The listing builds one solid part. Answer for the finished solid, in the listing's coordinates (mm). A direction names the side the tool comes from. Give positions to 0.01 mm unless a question says otherwise; leave off trailing zeros. Order: outer loops, then holes, each group sorted by start corner. A loop starts at its lowest first (then second) coordinate and runs counter-clockwise, first axis right, second up. Notation, with made-up numbers: (9.25, 63.25) -> (36.25, 63.25) arc R21 ccw to (36.25, 69.25) -> close; hole circle Ø10 at (-8.5, -26.5). An arc over 180 degrees is marked (long way). One line per question, with ' | ' between items. Start each with the question number.
```python
from build123d import *

# Parameters (mm, degrees)
BASE_FLANGE_DEPTH               = 1.5875
EDGE_FLANGE1_STRIP_W            = 7.8232
EDGE_FLANGE1_STRIP_H            = 1.5875
EDGE_FLANGE1_STRIP_CUT_DEPTH    = 139.7
EDGE_FLANGE1_DEPTH              = 139.7
EDGE_FLANGE2_STRIP_W            = 7.8232
EDGE_FLANGE2_STRIP_H            = 1.5875
EDGE_FLANGE2_STRIP_CUT_DEPTH    = 139.7
EDGE_FLANGE2_DEPTH              = 139.7
EDGE_FLANGE3_STRIP_W            = 7.8232
EDGE_FLANGE3_STRIP_H            = 1.5875
EDGE_FLANGE3_STRIP_CUT_DEPTH    = 370.68125
EDGE_FLANGE3_DEPTH              = 370.68125
EDGE_FLANGE4_STRIP_W            = 7.8232
EDGE_FLANGE4_STRIP_H            = 1.5875
EDGE_FLANGE4_STRIP_CUT_DEPTH    = 370.68125
EDGE_FLANGE4_DEPTH              = 370.68125
SKETCH15_W                      = 20.4724
SKETCH15_H                      = 10.668
CUT_EXTRUDE1_DEPTH              = 458.107468491
SKETCH16_W                      = 17.653
SKETCH16_H                      = 13.081
CUT_EXTRUDE2_DEPTH              = 458.107468491
F_1_8_0_125_DIAMETER_HOLE1_D    = 3.175
LPATTERN2_COUNT                 = 2
LPATTERN2_PITCH                 = 24.9936
SKETCH20_W                      = 17.145
SKETCH20_H                      = 22.987
CUT_EXTRUDE4_DEPTH              = 458.107468491
F_40_0_098_DIAMETER_HOLE2_D     = 3.175
SKETCH31_W                      = 30.48
SKETCH31_H                      = 22.86
CUT_EXTRUDE5_DEPTH              = 458.107468491
F_40_0_098_DIAMETER_HOLE3_D     = 3.556
F_40_0_098_DIAMETER_HOLE4_D     = 3.556
F_40_0_098_DIAMETER_HOLE4_DEPTH = 1.5875
F_40_0_098_DIAMETER_HOLE4_TIP   = 1.068330181
FILLET1_R                       = 5.9436
SKETCH38_W                      = 20.4724
SKETCH38_H                      = 10.668
CUT_EXTRUDE6_DEPTH              = 2.54
LPATTERN3_COUNT                 = 2
LPATTERN3_PITCH                 = 32.4866
LPATTERN4_COUNT                 = 2
LPATTERN4_PITCH                 = 24.9936
LPATTERN5_COUNT                 = 2
LPATTERN5_PITCH                 = 32.4866
LPATTERN7_COUNT                 = 2
LPATTERN7_PITCH                 = 57.4802
LPATTERN8_COUNT                 = 2
LPATTERN8_PITCH                 = 88.9
SKETCH41_R                      = 4.7117
CUT_EXTRUDE7_DEPTH              = 2.54
SKETCH43_W                      = 7.7978
SKETCH43_H                      = 4.0132
CUT_EXTRUDE8_DEPTH              = 2.54
HOLE1_START                     = -15.0368
HOLE1_OUTLINE_R                 = 2.7051
HOLE1_DEPTH                     = 169.7736
LPATTERN9_COUNT                 = 3
LPATTERN9_PITCH                 = 177.8


# Read off the part's stored shape, not the designer's step: Hole1
# Sheet-metal steps are written as plain solids
with BuildPart() as part:
    # Sketch1 → Base-Flange (new body)
    with BuildSketch(Plane.XY):
        Polygon((0, 0), (28.832175, 0), (28.832175, -13.4493), (399.513425, -13.4493), (399.513425, 0), (428.3456, 0), (428.3456, 139.7), (399.513425, 139.7), (399.513425, 153.1493), (28.832175, 153.1493), (28.832175, 139.7), (0, 139.7), align=None)
    extrude(amount=BASE_FLANGE_DEPTH)

    # Edge-Flange1 strip (across the edge) → Edge-Flange1 strip cut (cut)
    with BuildSketch(Plane(origin=(428.3456, 0, 1.5875), x_dir=(-1, 0, 0), z_dir=(0, 1, 0))):
        with Locations((-3.175, -0.79375)):
            Rectangle(EDGE_FLANGE1_STRIP_W, EDGE_FLANGE1_STRIP_H)
    extrude(amount=EDGE_FLANGE1_STRIP_CUT_DEPTH, mode=Mode.SUBTRACT)

    # Edge-Flange1 section (across the edge) → Edge-Flange1 (add)
    with BuildSketch(Plane(origin=(428.3456, 0, 1.5875), x_dir=(-1, 0, 0), z_dir=(0, 1, 0))):
        with BuildLine():
            Line((-1.5875, 0.7366), (-1.5875, 12.7))
            Line((-1.5875, 12.7), (0, 12.7))
            Line((0, 12.7), (0, 0.7366))
            ThreePointArc((0, 0.7366), (0.215745145, 0.215745145), (0.7366, 0))
            Line((0.7366, 0), (0.7366, -1.5875))
            ThreePointArc((0.7366, -1.5875), (-0.90678687, -0.90678687), (-1.5875, 0.7366))
        make_face()
    extrude(amount=EDGE_FLANGE1_DEPTH)

    # Edge-Flange2 strip (across the edge) → Edge-Flange2 strip cut (cut)
    with BuildSketch(Plane(origin=(0, 139.7, 1.5875), x_dir=(1, 0, 0), z_dir=(0, -1, 0))):
        with Locations((-3.175, -0.79375)):
            Rectangle(EDGE_FLANGE2_STRIP_W, EDGE_FLANGE2_STRIP_H)
    extrude(amount=EDGE_FLANGE2_STRIP_CUT_DEPTH, mode=Mode.SUBTRACT)

    # Edge-Flange2 section (across the edge) → Edge-Flange2 (add)
    with BuildSketch(Plane(origin=(0, 139.7, 1.5875), x_dir=(1, 0, 0), z_dir=(0, -1, 0))):
        with BuildLine():
            Line((-1.5875, 0.7366), (-1.5875, 12.7))
            Line((-1.5875, 12.7), (0, 12.7))
            Line((0, 12.7), (0, 0.7366))
            ThreePointArc((0, 0.7366), (0.215745145, 0.215745145), (0.7366, 0))
            Line((0.7366, 0), (0.7366, -1.5875))
            ThreePointArc((0.7366, -1.5875), (-0.90678687, -0.90678687), (-1.5875, 0.7366))
        make_face()
    extrude(amount=EDGE_FLANGE2_DEPTH)

    # Edge-Flange3 strip (across the edge) → Edge-Flange3 strip cut (cut)
    with BuildSketch(Plane(origin=(399.513425, 153.1493, 1.5875), x_dir=(0, -1, 0), z_dir=(-1, 0, 0))):
        with Locations((-3.175, -0.79375)):
            Rectangle(EDGE_FLANGE3_STRIP_W, EDGE_FLANGE3_STRIP_H)
    extrude(amount=EDGE_FLANGE3_STRIP_CUT_DEPTH, mode=Mode.SUBTRACT)

    # Edge-Flange3 section (across the edge) → Edge-Flange3 (add)
    with BuildSketch(Plane(origin=(399.513425, 153.1493, 1.5875), x_dir=(0, -1, 0), z_dir=(-1, 0, 0))):
        with BuildLine():
            Line((-1.5875, 0.7366), (-1.5875, 12.7))
            Line((-1.5875, 12.7), (0, 12.7))
            Line((0, 12.7), (0, 0.7366))
            ThreePointArc((0, 0.7366), (0.215745145, 0.215745145), (0.7366, 0))
            Line((0.7366, 0), (0.7366, -1.5875))
            ThreePointArc((0.7366, -1.5875), (-0.90678687, -0.90678687), (-1.5875, 0.7366))
        make_face()
    extrude(amount=EDGE_FLANGE3_DEPTH)

    # Edge-Flange4 strip (across the edge) → Edge-Flange4 strip cut (cut)
    with BuildSketch(Plane(origin=(28.832175, -13.4493, 1.5875), x_dir=(0, 1, 0), z_dir=(1, 0, 0))):
        with Locations((-3.175, -0.79375)):
            Rectangle(EDGE_FLANGE4_STRIP_W, EDGE_FLANGE4_STRIP_H)
    extrude(amount=EDGE_FLANGE4_STRIP_CUT_DEPTH, mode=Mode.SUBTRACT)

    # Edge-Flange4 section (across the edge) → Edge-Flange4 (add)
    with BuildSketch(Plane(origin=(28.832175, -13.4493, 1.5875), x_dir=(0, 1, 0), z_dir=(1, 0, 0))):
        with BuildLine():
            Line((-1.5875, 0.7366), (-1.5875, 12.7))
            Line((-1.5875, 12.7), (0, 12.7))
            Line((0, 12.7), (0, 0.7366))
            ThreePointArc((0, 0.7366), (0.215745145, 0.215745145), (0.7366, 0))
            Line((0.7366, 0), (0.7366, -1.5875))
            ThreePointArc((0.7366, -1.5875), (-0.90678687, -0.90678687), (-1.5875, 0.7366))
        make_face()
    extrude(amount=EDGE_FLANGE4_DEPTH)

    # Sketch15 → Cut-Extrude1 (cut, through all)
    with BuildSketch(Plane.XY.offset(1.5875)):
        with Locations((74.4728, 119.6213)):
            Rectangle(SKETCH15_W, SKETCH15_H)
    extrude(amount=-CUT_EXTRUDE1_DEPTH, mode=Mode.SUBTRACT)

    # Sketch16 → Cut-Extrude2 (cut, through all)
    with BuildSketch(Plane.XY.offset(1.5875)):
        with Locations((105.8291, 119.6213)):
            Rectangle(SKETCH16_W, SKETCH16_H)
    extrude(amount=-CUT_EXTRUDE2_DEPTH, mode=Mode.SUBTRACT)

    # 1/8 (0.125) Diameter Hole1 (through all)
    with Locations(Plane.XY.offset(1.5875)):
        with Locations((61.976, 119.6213)):
            f_1_8_0_125_diameter_hole1 = Hole(F_1_8_0_125_DIAMETER_HOLE1_D / 2)

    # LPattern2: 1/8 (0.125) Diameter Hole1 ×2
    with Locations(*[(i * LPATTERN2_PITCH, 0, 0) for i in range(1, LPATTERN2_COUNT)]):
        add(f_1_8_0_125_diameter_hole1, mode=Mode.SUBTRACT)

    # Sketch20 → Cut-Extrude4 (cut, through all)
    with BuildSketch(Plane.XY.offset(1.5875)):
        with Locations((42.9641, 119.6213)):
            Rectangle(SKETCH20_W, SKETCH20_H)
    extrude(amount=-CUT_EXTRUDE4_DEPTH, mode=Mode.SUBTRACT)

    # #40 (0.098) Diameter Hole2 (through all)
    with Locations(Plane.XY.offset(1.5875)):
        with Locations((42.9641, 134.1247), (42.9641, 105.1179)):
            Hole(F_40_0_098_DIAMETER_HOLE2_D / 2)

    # Sketch31 → Cut-Extrude5 (cut, through all)
    with BuildSketch(Plane.XY.offset(1.5875)):
        with Locations((394.3731, 21.7932)):
            Rectangle(SKETCH31_W, SKETCH31_H)
    extrude(amount=-CUT_EXTRUDE5_DEPTH, mode=Mode.SUBTRACT)

    # #40 (0.098) Diameter Hole3 (through all)
    with Locations(Plane(origin=(374.3706, 21.7932, 1.5875), x_dir=(1, 0, 0), z_dir=(0, 0, 1))):
        with Locations((0, 0)):
            Hole(F_40_0_098_DIAMETER_HOLE3_D / 2)

    # #40 (0.098) Diameter Hole4
    with Locations(Plane.XY.offset(1.5875)):
        with Locations((414.3756, 21.7932)):
            Hole(F_40_0_098_DIAMETER_HOLE4_D / 2, depth=F_40_0_098_DIAMETER_HOLE4_DEPTH)
            with Locations((0, 0, -(F_40_0_098_DIAMETER_HOLE4_DEPTH + F_40_0_098_DIAMETER_HOLE4_TIP / 2))):  # 118° drill point
                Cone(0, F_40_0_098_DIAMETER_HOLE4_D / 2, F_40_0_098_DIAMETER_HOLE4_TIP, mode=Mode.SUBTRACT)

    # Fillet1
    fillet1_edges = [part.edges().sort_by_distance(p)[0] for p in [
        (379.1331, 10.3632, 0.79375),
        (379.1331, 33.2232, 0.79375),
        (409.6131, 33.2232, 0.79375),
        (409.6131, 10.3632, 0.79375),
    ]]
    fillet(fillet1_edges, radius=FILLET1_R)

    # Sketch38 → Cut-Extrude6 (cut)
    with BuildSketch(Plane(origin=(0, 0, 0), x_dir=(-1, 0, 0), z_dir=(0, 0, -1))):
        with Locations((-230.779365766, 2.9972)):
            Rectangle(SKETCH38_W, SKETCH38_H)
    cut_extrude6 = extrude(amount=-CUT_EXTRUDE6_DEPTH, mode=Mode.SUBTRACT)

    # LPattern3: Cut-Extrude6 ×2
    with Locations(*[(-i * LPATTERN3_PITCH, 0, 0) for i in range(1, LPATTERN3_COUNT)]):
        add(cut_extrude6, mode=Mode.SUBTRACT)

    # Sketch39 → #40 (0.098) Diameter Hole5 (revolve, cut)
    with BuildSketch(Plane(origin=(243.276165766, 2.9972, 0), x_dir=(0, 1, 0), z_dir=(1, 0, 0))):
        Polygon((0, 0), (0, 4.090711583), (1.524, 3.175), (1.524, 0), align=None)
    f_40_0_098_diameter_hole5 = revolve(axis=Axis((243.276165766, 2.9972, -6.35), (0, 0, 1)), mode=Mode.SUBTRACT)

    # LPattern4: #40 (0.098) Diameter Hole5 ×2
    with Locations(*[(-i * LPATTERN4_PITCH, 0, 0) for i in range(1, LPATTERN4_COUNT)]):
        add(f_40_0_098_diameter_hole5, mode=Mode.SUBTRACT)

    # LPattern5: #40 (0.098) Diameter Hole5 ×2
    with Locations(*[(-i * LPATTERN5_PITCH, 0, 0) for i in range(1, LPATTERN5_COUNT)]):
        add(f_40_0_098_diameter_hole5, mode=Mode.SUBTRACT)

    # LPattern7: #40 (0.098) Diameter Hole5 ×2
    with Locations(*[(-i * LPATTERN7_PITCH, 0, 0) for i in range(1, LPATTERN7_COUNT)]):
        add(f_40_0_098_diameter_hole5, mode=Mode.SUBTRACT)

    # Sketch42 → CSK for #4 Flat Head Machine Screw1 (revolve, cut)
    with BuildSketch(Plane(origin=(429.9331, 114.3, 8.3058), x_dir=(0, 0, -1), z_dir=(0, 1, 0))):
        Polygon((0, 0), (0, 1.5885), (1.63195, 1.5885), (1.63195, 1.409834001), (2.8575, 0), align=None)
    csk_for_4_flat_head_machine_screw1 = revolve(axis=Axis((436.2831, 114.3, 8.3058), (-1, 0, 0)), mode=Mode.SUBTRACT)

    # LPattern8: CSK for #4 Flat Head Machine Screw1 ×2
    with Locations(*[(0, -i * LPATTERN8_PITCH, 0) for i in range(1, LPATTERN8_COUNT)]):
        add(csk_for_4_flat_head_machine_screw1, mode=Mode.SUBTRACT)

    # Mirror1: CSK for #4 Flat Head Machine Screw1 across plane
    add(csk_for_4_flat_head_machine_screw1.mirror(Plane.ZY.offset(-214.1728)), mode=Mode.SUBTRACT)

    # Mirror1 copy 1 sketch → Mirror1 copy 1 (revolve, cut)
    with BuildSketch(Plane(origin=(-1.5875, 25.4, 8.3058), x_dir=(0, 0, -1), z_dir=(0, 1, 0))):
        Polygon((0, 0), (0, -1.5885), (1.63195, -1.5885), (1.63195, -1.409834001), (2.8575, 0), align=None)
    revolve(axis=Axis((-7.9375, 25.4, 8.3058), (-1, 0, 0)), mode=Mode.SUBTRACT)

    # Sketch41 → Cut-Extrude7 (cut)
    with BuildSketch(Plane(origin=(0, 0, 0), x_dir=(-1, 0, 0), z_dir=(0, 0, -1))):
        with Locations((-90.588465, 2.813286828)):
            Circle(SKETCH41_R)
    extrude(amount=-CUT_EXTRUDE7_DEPTH, mode=Mode.SUBTRACT)

    # Sketch43 → Cut-Extrude8 (cut)
    with BuildSketch(Plane.XY.offset(1.5875)):
        with Locations((107.187365, -0.331233172)):
            Rectangle(SKETCH43_W, SKETCH43_H)
    extrude(amount=-CUT_EXTRUDE8_DEPTH, mode=Mode.SUBTRACT)

    # Hole1 outline → Hole1 (cut)
    with BuildSketch(Plane(origin=(0, 0, 0), x_dir=(1, 0, 0), z_dir=(0, 1, 0)).offset(HOLE1_START)):
        with Locations((33.0835, -8.6233)):
            Circle(HOLE1_OUTLINE_R)
    hole1 = extrude(amount=HOLE1_DEPTH, mode=Mode.SUBTRACT)

    # LPattern9: Hole1 ×3
    with Locations(*[(i * LPATTERN9_PITCH, 0, 0) for i in range(1, LPATTERN9_COUNT)]):
        add(hole1, mode=Mode.SUBTRACT)


solid = part.part
```
(1) For faces 5 (the face through (428.346, 69, 8)), 6 (the face through (217, 153.149, 8)), 7 (the face through (418, 0, 1)), 8 (the face through (28.832, -10, 1)), 9 (the face through (418, 139.7, 1)), determine the directions among +Z, -Z, +X, -X, +Y, -Y from which every point of the face is accessible in a straight line to the end or side of a thin tool.
(2) The part is cut by section A-A on x = 138. Determine the outline of the cut face in (y, z), plus the area to 3 significant figures.
(3) Consider line 1 (Y direction, x = 102.5, z = 8.25); line 2 (X direction, y = 70.5, z = 13.25); line 3 (Z direction, x = 85, y = 137). Determine where each line is inside the solid, lowest interval first.
(4) Determine the mould class of faces 1 (the face through (399.513, 150, 1)), 2 (the face through (211, 71, 1.588)), 3 (the face through (0, 71, 8)), 4 (the face through (10, 139.7, 1)) for opening direction X: pulls with the +X half, pulls with the -X half, needs draft (parallel to the pull), parting line crosses it, or undercut.
(5) Given P1, Ø7, axis at y = 149, z = 4.5, coming from the +X side; P2, Ø5, axis at x = 388.68, z = 8.62, coming from the +Y side; P3, Ø0.5, axis at y = 121, z = 0.5, coming from the -X side; P4, Ø3.5, axis at x = 243.28, y = 3, coming from the +Z side, each flat-ended and moving along its own axis, determine where each tip first touches the part or whether it passes through.
(6) The part is cut by section B-B on y = 93. Determine the outline of the cut face in (x, z).
Result sheet:
1) face 5: +Z, +Y, -Y | face 6: +Z, +X, -X | face 7: +Z, -Z, +X, -Y | face 8: +Z, -Z, -X, -Y | face 9: +Z, -Z, +X, +Y
2) outline: (-15.04, 2.32) arc R2.32 ccw to (-12.71, 0) -> (152.41, 0) arc R2.32 ccw to (154.74, 2.32) -> (154.74, 14.29) -> (153.15, 14.29) -> (153.15, 2.32) arc R0.74 cw to (152.41, 1.59) -> (-12.71, 1.59) arc R0.74 cw to (-13.45, 2.32) -> (-13.45, 14.29) -> (-15.04, 14.29) -> close | area: 308 mm^2
3) line 1: y = -15.04 to -13.45, 153.15 to 154.74 | line 2: x = -1.59 to 0, 428.35 to 429.93 | line 3: z = 0 to 1.59
4) face 1: pulls with the +X half | face 2: undercut | face 3: undercut | face 4: needs draft
5) P1: stops at x = 399.51 | P2: passes through | P3: stops at x = -0.97 | P4: stops at z = 1.59
6) outline: (-1.59, 2.32) arc R2.32 ccw to (0.74, 0) -> (427.61, 0) arc R2.32 ccw to (429.93, 2.32) -> (429.93, 14.29) -> (428.35, 14.29) -> (428.35, 2.32) arc R0.74 cw to (427.61, 1.59) -> (0.74, 1.59) arc R0.74 cw to (0, 2.32) -> (0, 14.29) -> (-1.59, 14.29) -> close
